from build123d import *

# Parameters (mm, degrees)
FILLET_R  = 2
PAD_DEPTH = 8


with BuildPart() as part:
    # Sketch → Revolution (revolve)
    with BuildSketch(Plane.XZ):
        with BuildLine():
            Line((0, 0), (20, 0))
            Line((20, 0), (20, 6))
            ThreePointArc((10, 16), (12.928932, 8.928932), (20, 6))
            Line((10, 16), (4, 16))
            Line((4, 16), (4, 52))
            Line((4, 52), (0, 52))
            Line((0, 52), (0, 0))
        make_face()
    revolve(axis=Axis((0, 0, 0), (0, 0, 1)))

    # Fillet
    fillet_edges = [part.edges().sort_by_distance(p)[0] for p in [
        (-10, 0, 16),
        (-20, 0, 6),
    ]]
    fillet(fillet_edges, radius=FILLET_R)

    # Sketch001 (on DatumPlane) → Pad (new body)
    with BuildSketch(Plane.XY.offset(19)):
        Polygon((3.752777, 6.5), (-3.752777, 6.5), (-7.505553, 0), (-3.752777, -6.5), (3.752777, -6.5), (7.505553, 0), align=None)
    extrude(amount=PAD_DEPTH)


solid = part.part
Verification items for the finished model (mm, model axes). A direction names the side the tool comes from. Round coordinates to 2 decimals unless told otherwise and drop trailing zeros. Order: outer loops, then holes, each group sorted by start corner. A loop starts at its lowest first (then second) coordinate and runs counter-clockwise, first axis right, second up. Notation, with made-up numbers: (75.25, 6) -> (120.25, 6) arc R32 cw to (120.25, 40) -> close; hole circle Ø5 at (12, 57). An arc over 180 degrees is marked (long way). Put each result on its own line as item: value.
1) Mould release check, pull along Z, two halves, no side actions. Record for faces 6 (the flat face through (3, -3, 27)), 7 (the flat face through (0, -6.5, 23)), 8 (the cylindrical face through (-0.867, -3.905, 17.521)), 9 (the flat face through (3, -3, 19)): +Z half, -Z half, draft (parallel to the pull), parting line (faces both ways), or undercut.
Final values:
face 6: +Z half
face 7: draft
face 8: undercut
face 9: undercut
2) Material ranges on line 1 (Z direction, x = 6.5, y = -1.5); line 2 (Z direction, x = 7.5, y = 2); line 3 (Z direction, x = 16, y = -7.5), recorded low to high.
Final values:
line 1: z = 0 to 16, 19 to 27
line 2: z = 0 to 16
line 3: z = 0 to 6.28
3) Depth check by flat-ended pin: pin 1 (6 mm diameter, centred on x = 7.5, z = 5.5, fed in from +Y); pin 2 (6 mm diameter, centred on x = -5, y = -14.5, fed in from +Z); pin 3 (1.5 mm diameter, centred on y = -1.5, z = 16.5, fed in from +X); pin 4 (12 mm diameter, centred on y = 11.5, z = 30.5, fed in from -X). Enter the tip coordinate at first touch or a pass-through.
Final values:
pin 1: stops at y = 19.42
pin 2: stops at z = 9.57
pin 3: stops at x = 9.02
pin 4: passes through
4) Set-up check for faces 1 (the flat face through (-5.66, -3.2, 22.94)), 2 (the flat face through (5.66, 3.2, 22.94)), 3 (the cylindrical face through (-0.867, -3.905, 39.675)), 4 (the flat face through (5.6, -3.3, 22.9)), 5 (the flat face through (4, -2, 16)): record each of +Z, -Z, +X, -X, +Y, -Y from which the full face is reachable in a straight line by a thin tool's end or side.
Final values:
face 1: +Z, -X, -Y
face 2: +Z, +X, +Y
face 3: +Z
face 4: +Z, +X, -Y
face 5: none
5) Section check A-A (z = 10.5). Record the cut outline in (x, y), then the cut area to 3 significant figures.
Final values:
outline: circle Ø23.3 at (0, 0)
area: 426 mm^2
